from build123d import *

# Parameters (mm, degrees)
SKETCH2_R           = 42.8622
SKETCH2_R_2         = 32.562372804
SKETCH2_R_3         = 1.524
BOSS_EXTRUDE1_DEPTH = 3.81
SKETCH3_R           = 42.8622
SKETCH3_R_2         = 40.3222
BOSS_EXTRUDE2_DEPTH = 44.45
SKETCH7_W           = 2.674266908
SKETCH7_H           = 10.16
SKETCH7_W_2         = 10.16
SKETCH7_H_2         = 2.674266908
CUT_EXTRUDE2_DEPTH  = 10.16
CUT_EXTRUDE3_DEPTH  = 10.16
SKETCH9_R           = 2.032
CUT_EXTRUDE4_DEPTH  = 10.16
CIRPATTERN2_COUNT   = 4
CUT_EXTRUDE5_DEPTH  = 78.481378264
CIRPATTERN3_COUNT   = 2
CIRPATTERN3_ANGLE   = 90


with BuildPart() as part:
    # Sketch2 → Boss-Extrude1 (new body)
    with BuildSketch(Plane.XY):
        with Locations(Location((0, 0, 0), (0, 0, 180))):
            Circle(SKETCH2_R)
        with Locations(Location((0, 0, 0), (0, 0, 180))):
            Circle(SKETCH2_R_2, mode=Mode.SUBTRACT)
        with Locations(Location((-19.05, 32.995567884, 0), (0, 0, 180))):
            Circle(SKETCH2_R_3, mode=Mode.SUBTRACT)
        with Locations(Location((-38.1, 0, 0), (0, 0, 180))):
            Circle(SKETCH2_R_3, mode=Mode.SUBTRACT)
        with Locations(Location((-19.05, -32.995567884, 0), (0, 0, 180))):
            Circle(SKETCH2_R_3, mode=Mode.SUBTRACT)
        with Locations(Location((19.05, -32.995567884, 0), (0, 0, 180))):
            Circle(SKETCH2_R_3, mode=Mode.SUBTRACT)
        with Locations(Location((38.1, 0, 0), (0, 0, 180))):
            Circle(SKETCH2_R_3, mode=Mode.SUBTRACT)
        with Locations(Location((19.05, 32.995567884, 0), (0, 0, 180))):
            Circle(SKETCH2_R_3, mode=Mode.SUBTRACT)
    extrude(amount=BOSS_EXTRUDE1_DEPTH)

    # Sketch3 → Boss-Extrude2 (add)
    with BuildSketch(Plane.XY.offset(3.81)):
        with Locations(Location((0, 0, 0), (0, 0, 180))):
            Circle(SKETCH3_R)
        Circle(SKETCH3_R_2, mode=Mode.SUBTRACT)
    extrude(amount=BOSS_EXTRUDE2_DEPTH)

    # Sketch7 → Cut-Extrude2 (cut)
    with BuildSketch(Plane.XY.offset(48.26)):
        with Locations((43.037064748, 0)):
            Rectangle(SKETCH7_W, SKETCH7_H)
        with Locations((0, -43.037064748)):
            Rectangle(SKETCH7_W_2, SKETCH7_H_2)
        with Locations((-43.037064748, 0)):
            Rectangle(SKETCH7_W, SKETCH7_H)
        with Locations((0, 43.037064748)):
            Rectangle(SKETCH7_W_2, SKETCH7_H_2)
    extrude(amount=-CUT_EXTRUDE2_DEPTH, mode=Mode.SUBTRACT)

    # Sketch8 → Cut-Extrude3 (cut)
    with BuildSketch(Plane(origin=(40.429931294, 0, 0), x_dir=(0, 0, -1), z_dir=(1, 0, 0))):
        Polygon((-38.604614587, 0), (-40.892307293, 3.9624), (-45.467692707, 3.9624), (-47.755385413, 0), (-45.467692707, -3.9624), (-40.892307293, -3.9624), align=None)
    cut_extrude3 = extrude(amount=-CUT_EXTRUDE3_DEPTH, mode=Mode.SUBTRACT)

    # Sketch9 → Cut-Extrude4 (cut)
    with BuildSketch(Plane(origin=(41.699931294, 0, 0), x_dir=(0, 0, -1), z_dir=(1, 0, 0))):
        with Locations((-43.18, 0)):
            Circle(SKETCH9_R)
    cut_extrude4 = extrude(amount=-CUT_EXTRUDE4_DEPTH, mode=Mode.SUBTRACT)

    # CirPattern2: Cut-Extrude3, Cut-Extrude4 ×4 about axis
    cirpattern2_axis = Axis((0, 0, 0), (0, 0, 1))
    add([cut_extrude3.rotate(cirpattern2_axis, i * 360 / CIRPATTERN2_COUNT) for i in range(1, CIRPATTERN2_COUNT)], mode=Mode.SUBTRACT)
    add([cut_extrude4.rotate(cirpattern2_axis, i * 360 / CIRPATTERN2_COUNT) for i in range(1, CIRPATTERN2_COUNT)], mode=Mode.SUBTRACT)

    # Sketch10 → Cut-Extrude5 (cut, symmetric)
    with BuildSketch(Plane(origin=(0, 0, 0), x_dir=(0, 0, 1), z_dir=(0.7071067811865464, 0.7071067811865488, 0))):
        with BuildLine():
            Line((7.547865198, 16.021870477), (7.547865198, 4.591870477))
            add(Edge.make_bspline(
                [(7.547865198, 4.591870477), (23.63247535, -7.228573119), (43.107865198, -11.410129523)],
                knots=[0, 0, 0, 1, 1, 1], degree=2))
            Line((43.107865198, -11.410129523), (43.107865198, 0.019870477))
            add(Edge.make_bspline(
                [(7.547865198, 16.021870477), (26.879831208, 11.531662429), (43.107865198, 0.019870477)],
                knots=[0, 0, 0, 1, 1, 1], degree=2))
        make_face()
    cut_extrude5 = extrude(amount=CUT_EXTRUDE5_DEPTH, both=True, mode=Mode.SUBTRACT)

    # CirPattern3: Cut-Extrude5 ×2 about axis
    cirpattern3_axis = Axis((0, 0, 48.26), (0, 0, 1))
    for i in range(1, CIRPATTERN3_COUNT):
        add(cut_extrude5.rotate(cirpattern3_axis, i * CIRPATTERN3_ANGLE / (CIRPATTERN3_COUNT - 1)), mode=Mode.SUBTRACT)


solid = part.part
The model under review builds one solid part; all positions refer to its coordinate system, in mm. A direction names the side the tool comes from. Round coordinates to 2 decimals unless told otherwise and drop trailing zeros. Loops run counter-clockwise (first coordinate to the right, second up) from the corner with the lowest first, then second, coordinate; pieces in that order, holes last. Notation, with made-up numbers: (8.5, 58.25) -> (59.5, 58.25) arc R24 ccw to (59.5, 89.25) -> close; hole circle Ø6 at (-12, 64). An arc over 180 degrees is marked (long way). Answer as CSV lines item,"result".
1) Tool access review of faces 3 (the face through (41.07, 0.61, 41.24)), 4 (the face through (41.7, -0.1, 41)), 5 (the face through (-41.7, -0.1, 41)), 6 (the face through (-36.577, -0.067, 1.878)), 7 (the face through (40.43, 2, 42)): name each direction out of +Z, -Z, +X, -X, +Y, -Y from which nothing blocks a thin tool from reaching the whole face with its end or side.
Geometry results:
face 3,"+X, -X"
face 4,"+Z, +X"
face 5,"+Z, -X"
face 6,"+Z, -Z"
face 7,"none"
2) Add section B-B on y = -11.5. Write out the cut boundary in (x, z), plus the area to 3 significant figures.
Geometry results:
outline,"(-41.29, 0) -> (-30.46, 0) -> (-30.46, 3.81) -> (-38.65, 3.81) -> (-38.65, 48.26) -> (-41.29, 48.26) -> close; (30.46, 0) -> (41.29, 0) -> (41.29, 48.26) -> (38.65, 48.26) -> (38.65, 3.81) -> (30.46, 3.81) -> close"
area,"317 mm²"
3) Add section D-D on z = 5.5. Write out the cut boundary in (x, y).
Geometry results:
outline,"circle Ø85.72 at (0, 0); hole circle Ø80.64 at (0, 0)"
4) Draft analysis for pull direction Y (two halves, no side actions). For faces 1 (the face through (18.23, 31.71, 1.88)), 2 (the face through (7, -32, 0)), state which applies: pulls with the +Y half, pulls with the -Y half, needs draft (parallel to the pull), parting line crosses it, or undercut.
Geometry results:
face 1,"undercut"
face 2,"needs draft"
5) To check wall thickness, follow line 1 along Y through (x, z) = (0, 20); line 2 along Z through (x, y) = (0, -41.25); line 3 along Y through (x, z) = (-19.05, 1.35). State the ranges of each line that lie inside material, in increasing order. Write a range as from..to.
Geometry results:
line 1,"y = -42.86..-40.32, 40.32..42.86"
line 2,"z = 0..41.15, 45.21..48.26"
line 3,"y = -38.4..-34.52, -31.47..-26.41, 26.41..31.47, 34.52..38.4"
6) For P1, Ø1.5, axis at x = -9.5, z = 14, coming from the -Y side; P2, Ø5, axis at y = -29, z = 37.5, coming from the +X side; P3, Ø3.5, axis at x = 0, z = 43.18, coming from the +Y side; P4, Ø9.5, axis at x = -31.5, y = -24.5, coming from the -Z side, all flat-tipped, find the tip position at first contact; note any pin that passes through.
Geometry results:
P1,"stops at y = -41.96"
P2,"stops at x = 33.69"
P3,"passes through"
P4,"stops at z = 0"
7) Add section A-A on x = -7. Write out the cut boundary in (y, z).
Geometry results:
outline,"(-42.29, 0) -> (-31.8, 0) -> (-31.8, 3.81) -> (-39.71, 3.81) -> (-39.71, 48.26) -> (-42.29, 48.26) -> close; (31.8, 0) -> (42.29, 0) -> (42.29, 48.26) -> (39.71, 48.26) -> (39.71, 3.81) -> (31.8, 3.81) -> close"
8) Add section C-C on z = 27.5. State how many separate pieces and enclosed holes the cut face has, plus the area to 3 significant figures.
Geometry results:
separate pieces,"4"
enclosed holes,"0"
area,"503 mm²"
